```python
from build123d import *

# Parameters (mm, degrees)
BOSS_EXTRUDE1_DEPTH = 1.2
EXTRUDE_THIN1_DEPTH = 1.2


with BuildPart() as part:
    # Sketch2 → Boss-Extrude1 (new body)
    with BuildSketch(Plane(origin=(0, 0, 0), x_dir=(1, 0, 0), z_dir=(0, 1, 0))):
        with BuildLine():
            Line((-4, 52.659282183), (-4, 49))
            ThreePointArc((-4, 49), (0, 45), (4, 49))
            Line((4, 49), (4, 52.659282183))
            ThreePointArc((4, 52.659282183), (4.668239922, 54.151399837), (6.226415094, 54.646424907))
            ThreePointArc((6.226415094, 54.646424907), (47.631397208, 27.5), (50.438399742, -21.930978807))
            ThreePointArc((50.438399742, -21.930978807), (49.23060787, -23.032885555), (47.604276115, -22.865539476))
            Line((47.604276115, -22.865539476), (44.435244785, -21.035898385))
            ThreePointArc((44.435244785, -21.035898385), (38.97114317, -22.5), (40.435244785, -27.964101615))
            Line((40.435244785, -27.964101615), (43.604276115, -29.793742707))
            ThreePointArc((43.604276115, -29.793742707), (44.562367948, -31.118514282), (44.211984648, -32.7154461))
            ThreePointArc((44.211984648, -32.7154461), (0, -55), (-44.211984648, -32.715446099))
            ThreePointArc((-44.211984648, -32.715446099), (-44.562367948, -31.118514282), (-43.604276115, -29.793742706))
            Line((-43.604276115, -29.793742706), (-40.435244785, -27.964101615))
            ThreePointArc((-40.435244785, -27.964101615), (-38.97114317, -22.5), (-44.435244785, -21.035898385))
            Line((-44.435244785, -21.035898385), (-47.604276115, -22.865539476))
            ThreePointArc((-47.604276115, -22.865539476), (-49.23060787, -23.032885555), (-50.438399742, -21.930978807))
            ThreePointArc((-50.438399742, -21.930978807), (-47.631397208, 27.5), (-6.226415094, 54.646424907))
            ThreePointArc((-6.226415094, 54.646424907), (-4.668239922, 54.151399837), (-4, 52.659282183))
        make_face()
    extrude(amount=BOSS_EXTRUDE1_DEPTH)

    # Sketch3 → Extrude-Thin1 (add)
    with BuildSketch(Plane.XZ):
        with BuildLine():
            ThreePointArc((-6.016981132, -52.808317887), (-5.900117994, -52.771191007), (-5.85, -52.659282183))
            Line((-5.85, -52.659282183), (-5.85, -49))
            ThreePointArc((-5.85, -49), (0, -43.15), (5.85, -49))
            Line((5.85, -49), (5.85, -52.659282183))
            ThreePointArc((5.85, -52.659282183), (5.900117994, -52.771191007), (6.016981132, -52.808317887))
            ThreePointArc((6.016981132, -52.808317887), (46.029250211, -26.575), (48.741835387, 21.193300429))
            ThreePointArc((48.741835387, 21.193300429), (48.651250997, 21.275943435), (48.529276115, 21.263392479))
            Line((48.529276115, 21.263392479), (45.360244785, 19.433751388))
            ThreePointArc((45.360244785, 19.433751388), (37.368996173, 21.575), (39.510244785, 29.566248612))
            Line((39.510244785, 29.566248612), (42.679276115, 31.395889704))
            ThreePointArc((42.679276115, 31.395889704), (42.751133003, 31.495247572), (42.724854255, 31.615017458))
            ThreePointArc((42.724854255, 31.615017458), (0, 53.15), (-42.724854255, 31.615017458))
            ThreePointArc((-42.724854255, 31.615017458), (-42.751133003, 31.495247572), (-42.679276115, 31.395889703))
            Line((-42.679276115, 31.395889703), (-39.510244785, 29.566248612))
            ThreePointArc((-39.510244785, 29.566248612), (-37.368996173, 21.575), (-45.360244785, 19.433751388))
            Line((-45.360244785, 19.433751388), (-48.529276115, 21.263392479))
            ThreePointArc((-48.529276115, 21.263392479), (-48.651250997, 21.275943435), (-48.741835387, 21.193300429))
            ThreePointArc((-48.741835387, 21.193300429), (-46.029250211, -26.575), (-6.016981132, -52.808317887))
        make_face()
        with BuildLine():
            Line((-7.45, -51.008822766), (-7.45, -49))
            ThreePointArc((-7.45, -49), (0, -41.55), (7.45, -49))
            Line((7.45, -49), (7.45, -51.008822766))
            ThreePointArc((7.45, -51.008822766), (44.643609565, -25.775), (47.899936333, 19.052522125))
            Line((47.899936333, 19.052522125), (46.160244785, 18.048110742))
            ThreePointArc((46.160244785, 18.048110742), (35.983355527, 20.775), (38.710244785, 30.951889258))
            Line((38.710244785, 30.951889258), (40.449936333, 31.956300641))
            ThreePointArc((40.449936333, 31.956300641), (0, 51.55), (-40.449936333, 31.956300641))
            Line((-40.449936333, 31.956300641), (-38.710244785, 30.951889258))
            ThreePointArc((-38.710244785, 30.951889258), (-35.983355527, 20.775), (-46.160244785, 18.048110742))
            Line((-46.160244785, 18.048110742), (-47.899936333, 19.052522125))
            ThreePointArc((-47.899936333, 19.052522125), (-44.643609565, -25.775), (-7.45, -51.008822766))
        make_face(mode=Mode.SUBTRACT)
    extrude(amount=EXTRUDE_THIN1_DEPTH)


solid = part.part
```
CAD build for the part. Positions are in the model's coordinates, mm. A direction names the side the tool comes from. Round coordinates to 2 decimals unless told otherwise and drop trailing zeros. Write each loop counter-clockwise with the first axis right and the second up, starting at its lowest first coordinate (ties: lowest second). Pieces come first, ordered by that corner, then holes. Notation, with made-up numbers: (44.25, 24.25) - (73.25, 24.25) arc R20 ccw to (73.25, 52.25) - close; hole circle Ø3 at (-4.5, 60.5). An arc over 180 degrees is marked (long way). Return JSON: item names as keys, results as strings. Group by question number.
Item 1: Flat gauge pins, fed straight in: pin 1 Ø1 at (y, z) = (0.5, -50.5) entering from +X; pin 2 Ø1 at (x, y) = (13, 0.5) entering from +Z; pin 3 Ø8 at (x, z) = (1, -11) entering from -Y. Where does each tip first touch, or does it go through?
Item 2: Band-saw the part on C-C on x = 0. List the corners of the cut face in (y, z).
Item 3: Mould opens along Z. For faces 1 (the face through (0.695, -0.592, 53.145)), 2 (the face through (-46.373, -0.592, -25.971)), 3 (the face through (36.07, -0.59, 20.63)), 4 (the face through (-0.2, -1.2, -42.8)) say: +Z half, -Z half, draft (parallel to the pull), parting line (faces both ways), or undercut.
Item 4: Probe probe 1 along Z at (x, y) = (40, -0.7); probe 2 along Y at (x, z) = (-21.5, -29); probe 3 along Z at (x, y) = (16, -0.1). List the from-to ranges inside material, lowest first.
Item 5: Band-saw the part on B-B on z = 24.5. List the corners of the cut face in (x, y).
Item 6: 3-axis set-ups, long thin cutter, end or side, ignore diameter. For faces 5 (the face through (-0.13, -0.59, -43.15)), 6 (the face through (-47.987, 0.592, -26.875)), 7 (the face through (1, 0, 0)), 8 (the face through (45.68, -0.59, -27.17)): which of +Z, -Z, +X, -X, +Y, -Y reach the whole face in a straight line?
Resolved:
{
 "1": {"pin 1": "stops at x = 22.91", "pin 2": "stops at z = 53.56", "pin 3": "stops at y = 0"},
 "2": {"outline": "(-1.2, -43.15) - (0, -43.15) - (0, -45) - (1.2, -45) - (1.2, 55) - (0, 55) - (0, 53.15) - (-1.2, 53.15) - (-1.2, 51.55) - (0, 51.55) - (0, -41.55) - (-1.2, -41.55) - close"},
 "3": {"face 1": "+Z half", "face 2": "parting line", "face 3": "undercut", "face 4": "draft"},
 "4": {"probe 1": "z = -35 to -32.52, 17.46 to 19.18, 29.85 to 31.7, 32.52 to 35", "probe 2": "y = 0 to 1.2", "probe 3": "z = -50.68 to -49, 49 to 50.68"},
 "5": {"outline": "(-38.44, 0) - (-36.59, 0) - (-36.59, -1.2) - (-34.99, -1.2) - (-34.99, 0) - (34.99, 0) - (34.99, -1.2) - (36.59, -1.2) - (36.59, 0) - (38.44, 0) - (38.44, 1.2) - (-38.44, 1.2) - close"},
 "6": {"face 5": "-Z, -Y", "face 6": "-X, +Y, -Y", "face 7": "-Y", "face 8": "+X, -Y"}
}
